```python
from build123d import *

# Parameters (mm, degrees)
SKETCH1_R           = 1.6
BOSS_EXTRUDE1_DEPTH = 6


with BuildPart() as part:
    # Sketch1 → Boss-Extrude1 (new body)
    with BuildSketch(Plane.XY):
        Polygon((6, 269), (106.875, 269), (106.875, 275), (116.875, 275), (116.875, 269), (215, 269), (215, 275), (225, 275), (225, 269), (323.125, 269), (323.125, 275), (333.125, 275), (333.125, 269), (434, 269), (434, 244), (440, 244), (440, 234), (434, 234), (434, 184), (440, 184), (440, 174), (434, 174), (434, 149), (333.125, 149), (333.125, 143), (323.125, 143), (323.125, 149), (225, 149), (225, 143), (215, 143), (215, 149), (116.875, 149), (116.875, 143), (106.875, 143), (106.875, 149), (6, 149), (6, 174), (0, 174), (0, 184), (6, 184), (6, 234), (0, 234), (0, 244), (6, 244), align=None)
        with Locations((111.875, 146)):
            Circle(SKETCH1_R, mode=Mode.SUBTRACT)
        with Locations((220, 146)):
            Circle(SKETCH1_R, mode=Mode.SUBTRACT)
        with Locations((328.125, 146)):
            Circle(SKETCH1_R, mode=Mode.SUBTRACT)
        with Locations((328.125, 272)):
            Circle(SKETCH1_R, mode=Mode.SUBTRACT)
        with Locations((220, 272)):
            Circle(SKETCH1_R, mode=Mode.SUBTRACT)
        with Locations((111.875, 272)):
            Circle(SKETCH1_R, mode=Mode.SUBTRACT)
        with Locations((3, 239)):
            Circle(SKETCH1_R, mode=Mode.SUBTRACT)
        with Locations((3, 179)):
            Circle(SKETCH1_R, mode=Mode.SUBTRACT)
        with Locations((437, 239)):
            Circle(SKETCH1_R, mode=Mode.SUBTRACT)
        with Locations((437, 179)):
            Circle(SKETCH1_R, mode=Mode.SUBTRACT)
    extrude(amount=-BOSS_EXTRUDE1_DEPTH)


solid = part.part
```
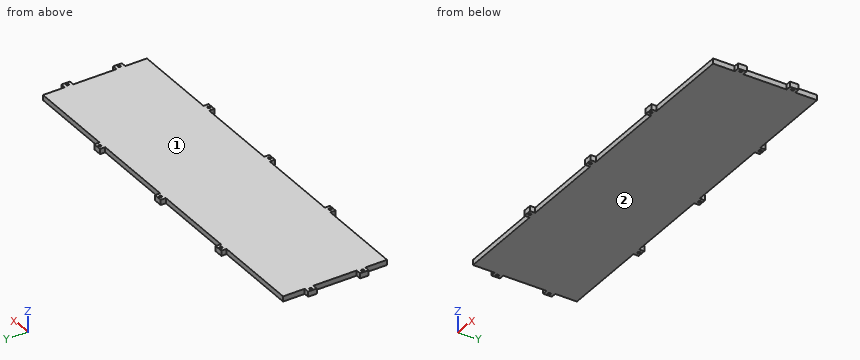
Input: part model. Units: mm. Frame: model coordinates. Face numbers are marked on the shaded views. Coordinates: 2 decimals unless noted, no trailing zeros. Write each loop counter-clockwise with the first axis right and the second up, starting at its lowest first coordinate (ties: lowest second). Pieces come first, ordered by that corner, then holes.
1) Section C-C on x = 408. Output: boundary loops of the cut face in (y, z), and give its area (3 significant figures).
2) Pin query (flat end, axial travel): pin 1 Ø2.5 at (x, y) = (220, 146) entering from -Z; pin 2 Ø1.8 at (x, z) = (271, -4) entering from +Y; pin 3 Ø3 at (x, z) = (250.5, -2.5) entering from -Y; pin 4 Ø1.8 at (x, z) = (3, -4.5) entering from +Y. Return the tip coordinate at first contact, or that it passes through.
3) Section B-B on y = 262. Output: boundary loops of the cut face in (x, z).
4) Mould query, pull axis Z, two halves, no side actions, for the marked faces 1 and 2. Classes: pulls with the +Z half, pulls with the -Z half, needs draft (parallel to the pull), parting line crosses it, or undercut.
5) Section A-A on z = -1.3. State how many separate pieces and enclosed holes the cut face has, and give its area (3 significant figures).
6) Material intervals for line 1 along X through (y, z) = (179, -3.1); line 2 along X through (y, z) = (272, -3.2) (3 decimals); line 3 along Y through (x, z) = (220, -1.65), sorted ascending.
Check result:
1. outline: (149, -6) - (269, -6) - (269, 0) - (149, 0) - close
1. area: 720 mm2
2. pin 1: passes through
2. pin 2: stops at y = 269
2. pin 3: stops at y = 149
2. pin 4: stops at y = 244
3. outline: (6, -6) - (434, -6) - (434, 0) - (6, 0) - close
4. face 1: pulls with the +Z half
4. face 2: pulls with the -Z half
5. separate pieces: 1
5. enclosed holes: 10
5. area: 51,900 mm2
6. line 1: x = 0 to 1.4, 4.6 to 435.4, 438.6 to 440
6. line 2: x = 106.875 to 110.275, 113.475 to 116.875, 215 to 218.4, 221.6 to 225, 323.125 to 326.525, 329.725 to 333.125
6. line 3: y = 143 to 144.4, 147.6 to 270.4, 273.6 to 275
